Here's the drawing with two shaded views (mm, measured from the low corner). I have some questions. Round coordinates to 2 decimals unless told otherwise and drop trailing zeros. Write each loop counter-clockwise with the first axis right and the second up, starting at its lowest first coordinate (ties: lowest second). Pieces come first, ordered by that corner, then holes. Notation, with made-up numbers: M -20.5,-18 L 4.5,-18 A6 cw 4.5,-14 Z; hole C 40,-1 d9. An arc over 180 degrees is marked long. Answer as a JSON object with one key per item and string values. Group by question number.
1) I'm going to push flat-ended pins straight in: pin 1 Ø1 at (y, z) = (4.5, 22.5) entering from +X; pin 2 Ø1.5 at (x, y) = (22.5, 3.5) entering from -Z; pin 3 Ø1.5 at (y, z) = (2.5, 37) entering from +X; pin 4 Ø8 at (x, z) = (16.51, 55.88) entering from +Y. Where does each tip first touch, or does it pass through?
2) Suppose I cut it at A-A, the plane y = 3. Write out the boundary of the cut face in (x, z).
3) If we mould it in two halves opening along X, with no side actions, what happens to the marked faces 1 and 2? For each: +X half, -X half, draft (parallel to the pull), parting line (faces both ways), or undercut.
4) Please list where these lines run through material, in increasing order: L1, parallel to X at y = 3.55, z = 25.4; L2, parallel to X at y = 2.4, z = 55.88 (1 decimal); L3, parallel to X at y = 3.05, z = 60. Write a range as [from, to].
5) Suppose I cut it at D-D, the plane z = 55.88. Write out the boundary of the cut face in (x, y), and give its area (3 significant figures).
6) Suppose I cut it at C-C, the plane x = 30.48. Write out the boundary of the cut face in (y, z).
7) Suppose I cut it at B-B, the plane z = 26. Write out the boundary of the cut face in (x, y) (1 decimal).
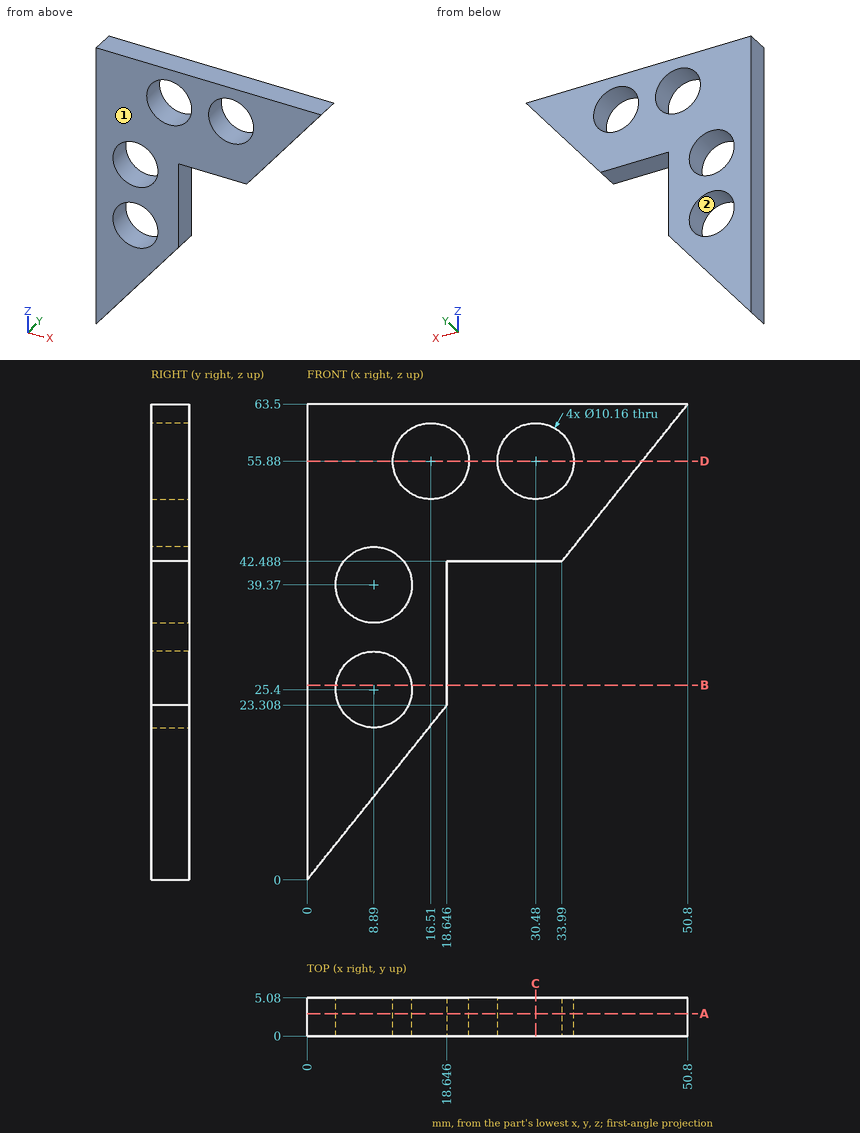
Results:
{
 "1": {"pin 1": "x = 18.4", "pin 2": "z = 42.49", "pin 3": "x = 18.65", "pin 4": "through"},
 "2": {"outline": "M 0,0 L 18.65,23.31 L 18.65,42.49 L 33.99,42.49 L 50.8,63.5 L 0,63.5 Z; hole C 8.89,25.4 d10.16; hole C 8.89,39.37 d10.16; hole C 16.51,55.88 d10.16; hole C 30.48,55.88 d10.16"},
 "3": {"face 1": "draft", "face 2": "undercut"},
 "4": {"L1": "[0, 3.81], [13.97, 18.65]", "L2": "[0, 11.4], [21.6, 25.4], [35.6, 44.7]", "L3": "[0, 13.54], [19.48, 27.51], [33.45, 48]"},
 "5": {"outline": "M 0,0 L 11.43,0 L 11.43,5.08 L 0,5.08 Z; M 21.59,0 L 25.4,0 L 25.4,5.08 L 21.59,5.08 Z; M 35.56,0 L 44.7,0 L 44.7,5.08 L 35.56,5.08 Z", "area": "124 mm^2"},
 "6": {"outline": "M 0,42.49 L 5.08,42.49 L 5.08,50.8 L 0,50.8 Z; M 0,60.96 L 5.08,60.96 L 5.08,63.5 L 0,63.5 Z"},
 "7": {"outline": "M 0,0 L 3.8,0 L 3.8,5.1 L 0,5.1 Z; M 13.9,0 L 18.6,0 L 18.6,5.1 L 13.9,5.1 Z"}
}
